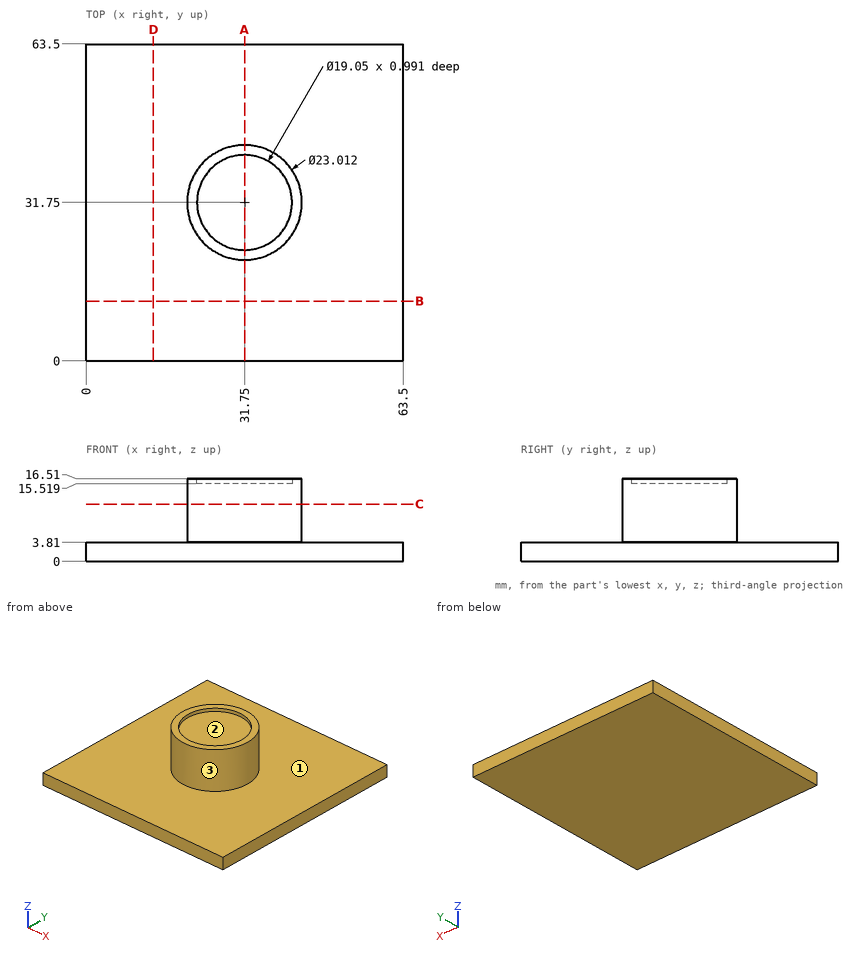
Print and shaded views of the part. All mm, measured from the part's lowest x, y and z. Coordinates: 2 decimals unless noted, no trailing zeros. Write each loop counter-clockwise with the first axis right and the second up, starting at its lowest first coordinate (ties: lowest second). Pieces come first, ordered by that corner, then holes.
(1) Cut at B-B, the plane y = 12. List the corners of the cut face in (x, z).
(2) Flat gauge pins, fed straight in: pin 1 (17 mm diameter, centred on x = 31.75, y = 31.75, fed in from +Z); pin 2 (1.5 mm diameter, centred on y = 43, z = 3.5, fed in from -X); pin 3 (6 mm diameter, centred on y = 24, z = 7, fed in from -X); pin 4 (2 mm diameter, centred on x = 48.5, y = 15, fed in from +Z). Where does each tip first touch, or does it go through?
(3) Drill centre lines: probe 1 along Y at (x, z) = (31.75, 16) (1 decimal); probe 2 along Z at (x, y) = (10.5, 55); probe 3 along X at (y, z) = (31.5, 6.25). Where is each one in solid material? Low to high.
(4) Cut at C-C, the plane z = 11.5. List the corners of the cut face in (x, y), and give its area (3 significant figures).
(5) Two-plate mould, pull along Y, no slides. Class the marked faces 1, 2 and 3: +Y half, -Y half, draft (parallel to the pull), parting line (faces both ways), or undercut.
(6) Cut at A-A, the plane x = 31.75. List the corners of the cut face in (y, z) (1 decimal).
Geometry says:
1. outline: (0, 0) - (63.5, 0) - (63.5, 3.81) - (0, 3.81) - close
2. pin 1: stops at z = 15.52
2. pin 2: stops at x = 0
2. pin 3: stops at x = 21.27
2. pin 4: stops at z = 3.81
3. probe 1: y = 20.2 to 22.2, 41.3 to 43.3
3. probe 2: z = 0 to 3.81
3. probe 3: x = 20.25 to 43.25
4. outline: circle Ø23.01 at (31.75, 31.75)
4. area: 416 mm2
5. face 1: draft
5. face 2: undercut
5. face 3: parting line
6. outline: (0, 0) - (63.5, 0) - (63.5, 3.8) - (43.3, 3.8) - (43.3, 16.5) - (41.3, 16.5) - (41.3, 15.5) - (22.2, 15.5) - (22.2, 16.5) - (20.2, 16.5) - (20.2, 3.8) - (0, 3.8) - close
